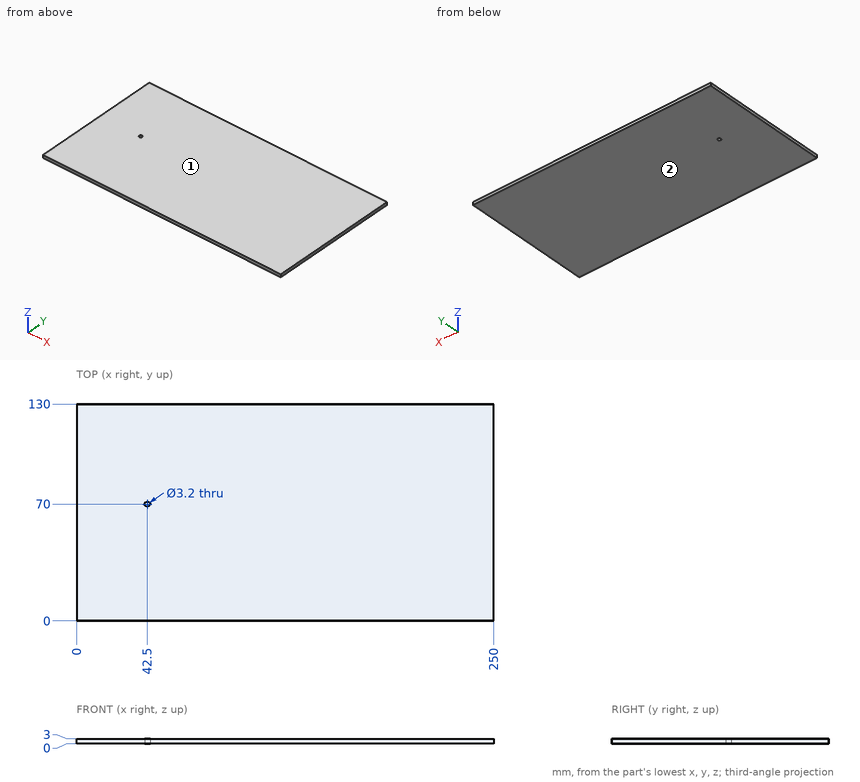
Part print with two shaded views. Sizes in mm from the minimum x, y, z corner. Coordinates: 2 decimals unless noted, no trailing zeros.
(1) Pin check, flat tips, straight feed: pin 1 Ø6 at (x, y) = (51, 16) entering from -Z; pin 2 Ø1.9 at (x, y) = (42.5, 70) entering from +Z. Stop position of each tip, or through.
(2) Mould opens along Z. For the marked faces 1 and 2 say: pulls with the +Z half, pulls with the -Z half, needs draft (parallel to the pull), parting line crosses it, or undercut.
(3) Drill centre lines: line 1 (Y direction, x = 42.5, z = 1.9); line 2 (X direction, y = 70, z = 1.3). Where is each one in solid material? Low to high.
Working result:
1. pin 1: stops at z = 0
1. pin 2: passes through
2. face 1: pulls with the +Z half
2. face 2: pulls with the -Z half
3. line 1: y = 0 to 68.4, 71.6 to 130
3. line 2: x = 0 to 40.9, 44.1 to 250
